```python
from build123d import *

# Parameters (mm, degrees)
F1_DEPTH = 4
F2_R     = 20
F3_R     = 19.99999


# Not quite as in the source:
# - a fillet or chamfer is up to 0.001 mm smaller than in the source, because OpenCascade refuses the exact size


with BuildPart() as f1:
    # F0 (on Top) → F1 (new body)
    with BuildSketch(Plane.XY):
        Polygon((0, 300), (0, 0), (150, 0), (150, 60), (130, 60), (130, 140), (90, 180), (130, 220), (130, 280), (110, 300), align=None)
        Polygon((150, 60), (150, 0), (300, 0), (300, 300), (190, 300), (170, 280), (170, 220), (210, 180), (170, 140), (170, 60), align=None)
    extrude(amount=F1_DEPTH)

    # F2
    f2_edges = [f1.edges().sort_by_distance(p)[0] for p in [
        (130, 60, 2),
        (130, 140, 2),
        (90, 180, 2),
        (130, 220, 2),
        (130, 280, 2),
        (110, 300, 2),
    ]]
    fillet(f2_edges, radius=F2_R)

    # F3 (radius 20 in the source; OpenCascade refuses exactly that, so slightly less here)
    f3_edges = [f1.edges().sort_by_distance(p)[0] for p in [
        (190, 300, 2),
        (170, 280, 2),
        (170, 220, 2),
        (210, 180, 2),
        (170, 140, 2),
        (170, 60, 2),
    ]]
    fillet(f3_edges, radius=F3_R)


solid = f1.part
```
Input: part model. Units: mm. Frame: model coordinates. A direction names the side the tool comes from. Give positions to 0.01 mm unless a question says otherwise; leave off trailing zeros. Loops run counter-clockwise (first coordinate to the right, second up) from the corner with the lowest first, then second, coordinate; pieces in that order, holes last.
1) Mould query, pull axis X, two halves, no side actions, for faces 4 (the flat face through (115, 152, 0)), 5 (the flat face through (114, 156, 2)). Classes: released by +X, released by -X, zero draft, split by the parting line, or undercut.
A:
face 4: zero draft
face 5: undercut
2) Contact query for a flat-ended pin moving along its axis: pin 1 (2 mm diameter, centred on x = 229, y = 105.5, fed in from -Z). Output: stop coordinate, or through.
A:
pin 1: stops at z = 0
3) Line query: L1, parallel to X at y = 256.5, z = 3.15; L2, parallel to X at y = 153, z = 1.6; L3, parallel to Y at x = 120.5, z = 1.15. Output: solid intervals per line, ascending.
A:
L1: x = 0 to 130, 170 to 300
L2: x = 0 to 117, 183 to 300
L3: y = 0 to 149.5, 210.5 to 289.5
4) Section query B-B on y = 149.5. Return the cut outline in (x, z), and give its area (3 significant figures).
A:
outline: (0, 0) - (120.5, 0) - (120.5, 4) - (0, 4) - close; (179.5, 0) - (300, 0) - (300, 4) - (179.5, 4) - close
area: 964 mm2
5) Reachability of faces 1 (the flat face through (115, 152, 4)), 2 (the flat face through (186, 204, 2)), 3 (the cylindrical face through (163.986, 65.703, 2.028)) from +Z, -Z, +X, -X, +Y, -Y: full face, straight path, thin tool, end or side. Return the list, or none.
A:
face 1: +Z, +X, -X, +Y, -Y
face 2: +Z, -Z
face 3: +Z, -Z, +Y
6) Section query D-D on x = 163. Return the cut outline in (y, z), and give its area (3 significant figures).
A:
outline: (0, 0) - (64.8, 0) - (64.8, 4) - (0, 4) - close
area: 259 mm2
7) Section query A-A on y = 242.5. Return the cut outline in (x, z), and give its area (3 significant figures).
A:
outline: (0, 0) - (130, 0) - (130, 4) - (0, 4) - close; (170, 0) - (300, 0) - (300, 4) - (170, 4) - close
area: 1,040 mm2
